Work out the finished part from the listing and answer in its coordinate system (mm). A direction names the side the tool comes from. Coordinates: 2 decimals unless noted, no trailing zeros. Order: outer loops, then holes, each group sorted by start corner. A loop starts at its lowest first (then second) coordinate and runs counter-clockwise, first axis right, second up. Notation, with made-up numbers: (49, 54) -> (80, 54) arc R24 cw to (80, 90) -> close; hole circle Ø7 at (87.5, 13). An arc over 180 degrees is marked (long way). Use one line per item in the form item = value.
Autodesk Inventor part; units mm, degrees
ref_plane "YZ Plane" through (0, 0, 0) normal (1, 0, 0) x (0, 1, 0)
ref_plane "XZ Plane" through (0, 0, 0) normal (0, 1, 0) x (-1, 0, 0)
ref_plane "XY Plane" through (0, 0, 0) normal (0, 0, 1) x (1, 0, 0)
sketch "Sketch1" plane through (0, 0, 0) normal (0, 1, 0) x (-1, 0, 0)
  circle A0 centre (-131.2765, -95.25) radius 3.3782
  circle A1 centre (-141.1255, -95.25) radius 3.3782
  circle A2 centre (-150.9745, -95.25) radius 3.3782
  circle A3 centre (-160.8235, -95.25) radius 3.3782
  line L0 (-146.05, -156.4252) -> (-146.05, 317.5689) construction
  line L1 (-125.73, -156.4252) -> (-125.73, 317.5689) construction
  line L2 (-166.37, -156.4252) -> (-166.37, 317.5689) construction
  line L3 (-166.37, -101.6) -> (-166.37, -76.2)
  line L4 (-166.37, -76.2) -> (-196.85, -76.2)
  line L5 (-196.85, -76.2) -> (-196.85, -50.8)
  line L6 (-196.85, -50.8) -> (-95.25, -50.8)
  line L7 (-95.25, -50.8) -> (-95.25, -76.2)
  line L8 (-95.25, -76.2) -> (-125.73, -76.2)
  line L9 (-125.73, -76.2) -> (-125.73, -101.6)
  line L10 (-166.37, -101.6) -> (-125.73, -101.6)
  dimension "d4" = 20.32
  dimension "d5" = 20.32
  dimension "d6" = 25.4
  dimension "d7" = 30.48
  dimension "d8" = 25.4
  dimension "d9" = 101.6
  dimension "d10" = 30.48
extrude "Extrusion1" add sketch "Sketch1" along normal blind 3.175
properties part number "Mount Motor"
(1) Section A-A on z = -95.25 is taken. Write down the section's boundary in (x, y) (3 decimals).
Data:
outline = (125.73, 0) -> (127.898, 0) -> (127.898, 3.175) -> (125.73, 3.175) -> close; (134.655, 0) -> (137.747, 0) -> (137.747, 3.175) -> (134.655, 3.175) -> close; (144.504, 0) -> (147.596, 0) -> (147.596, 3.175) -> (144.504, 3.175) -> close; (154.353, 0) -> (157.445, 0) -> (157.445, 3.175) -> (154.353, 3.175) -> close; (164.202, 0) -> (166.37, 0) -> (166.37, 3.175) -> (164.202, 3.175) -> close
(2) Which of the six approach directions +Z, -Z, +X, -X, +Y, -Y give full straight-line access (tool end or side, diameter ignored) to faces 1 (the flat face through (181, 2, -76.2)), 2 (the flat face through (125.73, 2, -89)), 3 (the flat face through (147, 0, -70))?
Data:
face_1 = -Z, +X, +Y, -Y
face_2 = -Z, -X, +Y, -Y
face_3 = +Z, -Z, +X, -X, -Y
(3) Section D-D on z = -81 is taken. Write down the section's boundary in (x, y) (3 decimals), plus the area to 3 significant figures.
Data:
outline = (125.73, 0) -> (166.37, 0) -> (166.37, 3.175) -> (125.73, 3.175) -> close
area = 129 mm²
(4) Section B-B on y = 1.4 is taken. Write down the section's boundary in (x, z), plus the area to 3 significant figures.
Data:
outline = (95.25, -76.2) -> (125.73, -76.2) -> (125.73, -101.6) -> (166.37, -101.6) -> (166.37, -76.2) -> (196.85, -76.2) -> (196.85, -50.8) -> (95.25, -50.8) -> close; hole circle Ø6.76 at (131.28, -95.25); hole circle Ø6.76 at (141.13, -95.25); hole circle Ø6.76 at (150.97, -95.25); hole circle Ø6.76 at (160.82, -95.25)
area = 3,470 mm²
(5) Each of these flat-tipped pins is pushed along its axis until it touches: P1, Ø1, axis at y = 1, z = -87, coming from the -X side; P2, Ø1.6, axis at x = 178.5, y = 1, coming from the -Z side. Where does it stop, or does it pass through?
Data:
P1 = 125.73
P2 = -76.2
(6) The mould has two halves that part along X. Classify faces 4 (the cylindrical face through (159.265, 1.565, -92.253)), 5 (the flat face through (95.25, 2, -63)), 6 (the flat face through (110, 2, -76.2)), 7 (the cylindrical face through (153.655, 1.565, -93.194)): released by +X, released by -X, zero draft, split by the parting line, or undercut.
Data:
face_4 = undercut
face_5 = released by -X
face_6 = zero draft
face_7 = undercut
(7) Section C-C on x = 183.5 is taken. Write down the section's boundary in (y, z) (3 decimals).
Data:
outline = (0, -76.2) -> (3.175, -76.2) -> (3.175, -50.8) -> (0, -50.8) -> close
(8) Straight lines are drawn through the part: line 1 along X through (y, z) = (0.7, -87.5); line 2 along X through (y, z) = (2.1, -93.5); line 3 along Z through (x, y) = (187.5, 3). For each, find the intervals that lie inside material, in ascending order.
Data:
line_1 = 125.73 to 166.37
line_2 = 125.73 to 128.39, 134.17 to 138.24, 144.02 to 148.08, 153.86 to 157.93, 163.71 to 166.37
line_3 = -76.2 to -50.8
